Design review of the part built by this model. Coordinates are the model's own, in mm. A direction names the side the tool comes from. Round coordinates to 2 decimals unless told otherwise and drop trailing zeros. Write each loop counter-clockwise with the first axis right and the second up, starting at its lowest first coordinate (ties: lowest second). Pieces come first, ordered by that corner, then holes. Notation, with made-up numbers: (48.5, 24.5) -> (73.5, 24.5) arc R8 cw to (73.5, 37.5) -> close; hole circle Ø8 at (73.5, -15.75). An arc over 180 degrees is marked (long way). One line per question, with ' | ' between items. Start each with the question number.
1) Mouldability with a two-part tool opening along Y and no side actions: class faces 4 (the cylindrical face through (-1.69, 12.89, 12.32)), 5 (the cylindrical face through (-3, 0, 3)), 6 (the flat face through (5.95, -9, 22)), 7 (the cylindrical face through (-3.238, 0.096, 6.106)) as +Y half, -Y half, draft (parallel to the pull), parting line (faces both ways), or undercut.
2) For probe 1 along Y at (x, z) = (0, 5); probe 2 along Y at (x, z) = (-0.5, 22.5), list the stretches that pass through material, from the lowest coordinate up.
3) Consider section A-A (y = -2.5). Give the boundary of the cut face in (x, z), then the cut area to 3 significant figures.
4) Insertion check: pin 1 Ø1.7 at (y, z) = (-9, 22) entering from +X; pin 2 Ø5 at (y, z) = (3, 15) entering from +X; pin 3 Ø6 at (x, z) = (-7.5, 22) entering from -Y; pin 4 Ø5 at (x, y) = (0, 0) entering from +Z. Each pin has a flat end and moves straight along its axis. Give the tip position at first contact, or say it passes through.
5) Consider section C-C (z = 17.5). Give the boundary of the cut face in (x, y), then the cut area to 3 significant figures.
6) Consider section B-B (x = 2.25). Give the boundary of the cut face in (y, z).
7) For faces 1 (the flat face through (0, 6.85, 15)), 2 (the flat face through (-3.45, -10, 22)), 3 (the flat face through (0, 9, 25)), list the 3-axis set-ups (+Z, -Z, +X, -X, +Y, -Y) from which the entire face can be reached by the end or side of a thin tool; tool diameter is ignored.
8) Consider section D-D (y = -6). Give the boundary of the cut face in (x, z).
```python
from build123d import *

# Parameters (mm, degrees)
SKETCH1_R               = 13
SKETCH1_R_2             = 3
BOSS_EXTRUDE1_DEPTH     = 25
CUT_EXTRUDE1_DEPTH      = 6.85
CUT_EXTRUDE2_REACH      = 33.032
CUT_EXTRUDE2_END_RADIUS = 13


with BuildPart() as part:
    # Sketch1 → Boss-Extrude1 (new body)
    with BuildSketch(Plane.XY):
        Circle(SKETCH1_R)
        Circle(SKETCH1_R_2, mode=Mode.SUBTRACT)
    extrude(amount=BOSS_EXTRUDE1_DEPTH)

    # Sketch2 → Cut-Extrude1 (cut, symmetric)
    with BuildSketch(Plane(origin=(0, 0, 0), x_dir=(1, 0, 0), z_dir=(0, 1, 0))):
        with BuildLine():
            Line((-6.8, -25), (6.8, -25))
            Line((6.8, -25), (6.8, -6.554936668))
            ThreePointArc((6.8, -6.554936668), (-0.224724758, -5.38457231), (-6.8, -8.119945437))
            Line((-6.8, -8.119945437), (-6.8, -25))
        make_face()
    extrude(amount=CUT_EXTRUDE1_DEPTH, both=True, mode=Mode.SUBTRACT)

    # Cut-Extrude2: up to this cylinder (the profile starts inside it)
    cut_extrude2_end = Plane(origin=(0, 0, 19.701869), z_dir=(0, 0, -1)) * Cylinder(CUT_EXTRUDE2_END_RADIUS, 93.064, mode=Mode.PRIVATE)
    # Sketch3 → Cut-Extrude2 (cut, up to the surface)
    with BuildSketch(Plane(origin=(0, 0, 0), x_dir=(1, 0, 0), z_dir=(0, 1, 0)), mode=Mode.PRIVATE) as cut_extrude2_sk1:
        with BuildLine():
            Line((-3.45, -18.2), (-3.45, -25))
            Line((-3.45, -25), (5.95, -25))
            Line((5.95, -25), (5.95, -18.2))
            ThreePointArc((5.95, -18.2), (1.25, -13.5), (-3.45, -18.2))
        make_face()
    cut_extrude2_tool1 = extrude(cut_extrude2_sk1.sketch, amount=-CUT_EXTRUDE2_REACH, mode=Mode.PRIVATE) & cut_extrude2_end
    add(cut_extrude2_tool1.solids().sort_by_distance((1.25, 0, 19.701869))[0], mode=Mode.SUBTRACT)


solid = part.part
```
From the geometry:
1) face 4: parting line | face 5: undercut | face 6: draft | face 7: undercut
2) probe 1: y = -13 to -3, 3 to 13 | probe 2: y = 6.85 to 12.99
3) outline: (-12.76, 0) -> (-1.66, 0) -> (-1.66, 5.63) arc R12.9 cw to (-6.8, 8.12) -> (-6.8, 25) -> (-12.76, 25) -> close; (1.66, 0) -> (12.76, 0) -> (12.76, 25) -> (6.8, 25) -> (6.8, 6.55) arc R12.9 cw to (1.66, 5.31) -> close | area: 362 mm2
4) pin 1: stops at x = 10.13 | pin 2: stops at x = 12.99 | pin 3: stops at y = -12.2 | pin 4: passes through
5) outline: (-6.8, -6.85) -> (-6.8, 6.85) -> (6.8, 6.85) -> (6.8, -6.85) -> (5.9, -6.85) -> (5.9, -11.59) arc R13 ccw (long way) to (-3.4, -12.55) -> (-3.4, -6.85) -> close | area: 291 mm2
6) outline: (-12.8, 0) -> (-1.98, 0) -> (-1.98, 5.34) -> (-6.85, 5.34) -> (-6.85, 13.61) -> (-12.8, 13.61) -> close; (1.98, 0) -> (12.8, 0) -> (12.8, 25) -> (6.85, 25) -> (6.85, 5.34) -> (1.98, 5.34) -> close
7) face 1: +Z | face 2: +Z, -Y | face 3: +Z, +X, -X, +Y, -Y
8) outline: (-11.53, 0) -> (11.53, 0) -> (11.53, 25) -> (6.8, 25) -> (6.8, 6.55) arc R12.9 cw to (-6.8, 8.12) -> (-6.8, 25) -> (-11.53, 25) -> close
